Geometry check sheet. Reference: the model listing, model coordinates, mm. Face numbers are marked on the shaded views. A direction names the side the tool comes from. Give positions to 0.01 mm unless a question says otherwise; leave off trailing zeros. Loops run counter-clockwise (first coordinate to the right, second up) from the corner with the lowest first, then second, coordinate; pieces in that order, holes last.
1. Cross-section at B-B, the plane z = 0. Record the cut outline in (x, y).
2. Go/stop test with flat-tipped pins: pin 1 Ø3 at (x, y) = (9, 2) entering from +Z; pin 2 Ø2.5 at (x, z) = (28, -1) entering from +Y; pin 3 Ø0.6 at (y, z) = (1.5, -5) entering from -X. Record where each tip stops, or that it passes through.
3. Tool access check on the marked faces 1, 2 and 3. Record the directions out of +Z, -Z, +X, -X, +Y, -Y that give a thin tool (end or side, any length) a straight path to the whole face; none if there is none.
4. Material ranges on L1, parallel to X at y = -1, z = 0.25; L2, parallel to Z at x = 18, y = 2.5; L3, parallel to Y at x = 10, z = 3.25, recorded low to high.
5. Cross-section at C-C, the plane y = 4. Record the cut outline in (x, z).
6. Release check for a two-part mould opening along X. For the marked faces 4, 5 and 6 record: +X half, -X half, draft (parallel to the pull), parting line (faces both ways), or undercut.
7. Cross-section at A-A, the plane x = 25. Record the cut outline in (y, z).
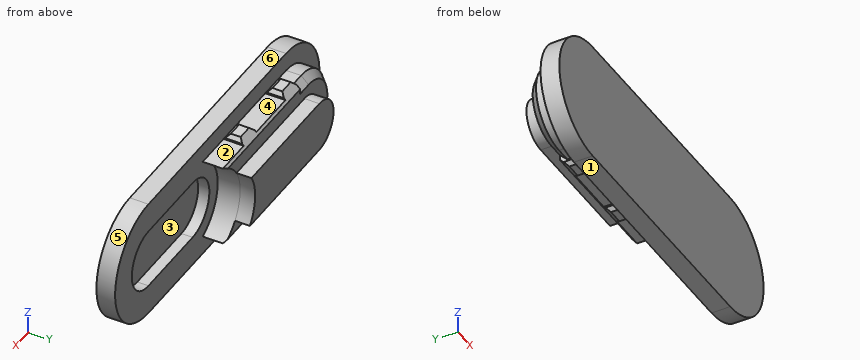
from build123d import *

# Parameters (mm, degrees)
EXTRUDE_1_DEPTH          = 3
EXTRUDE_2_DEPTH          = 2.5
CUT_EXTRUDE_1_DEPTH      = 1.5
EXTRUDE_3_DEPTH          = 2
SKETCH_5_W               = 3
SKETCH_5_H               = 0.7
EXTRUDE_4_DEPTH          = 3
CHAMFER_1_SIZE           = 1
CHAMFER_START            = -5.499796234
CHAMFER_2_DEPTH          = 7.499796234
CHAMFER_2_2_ANGLE        = 180
CHAMFER_3_SIZE           = 0.5
CUT_EXTRUDE_2_DEPTH      = 43.071367936
CUT_EXTRUDE_2_DEPTH_BACK = 43.071367936


with BuildPart() as part:
    # 草图1 → 凸台-拉伸1 (new body)
    with BuildSketch(Plane(origin=(0, 0, 0), x_dir=(1, 0, 0), z_dir=(0, 1, 0))):
        with BuildLine():
            Line((0, 5.5), (20.002084238, 5.5))
            ThreePointArc((20.002084238, 5.5), (16.4, 0), (20.002084238, -5.5))
            Line((20.002084238, -5.5), (0, -5.5))
            ThreePointArc((0, -5.5), (-5.5, 0), (0, 5.5))
        make_face()
    extrude(amount=EXTRUDE_1_DEPTH)

    # 草图2 → 凸台-拉伸2 (add)
    with BuildSketch(Plane.XZ):
        with BuildLine():
            Line((0, 8), (33, 8))
            ThreePointArc((33, 8), (41, 0), (33, -8))
            Line((33, -8), (0, -8))
            ThreePointArc((0, -8), (-8, 0), (0, 8))
        make_face()
    extrude(amount=EXTRUDE_2_DEPTH)

    # 草图3 → 切除-拉伸1 (cut)
    with BuildSketch(Plane(origin=(0, 0, 0), x_dir=(1, 0, 0), z_dir=(0, 1, 0))):
        with BuildLine():
            Line((22.4, 4), (33, 4))
            ThreePointArc((33, 4), (37, 0), (33, -4))
            Line((33, -4), (22.4, -4))
            ThreePointArc((22.4, -4), (18.4, 0), (22.4, 4))
        make_face()
    extrude(amount=-CUT_EXTRUDE_1_DEPTH, mode=Mode.SUBTRACT)

    # 草图4 → 凸台-拉伸3 (add)
    with BuildSketch(Plane(origin=(0, 3, 0), x_dir=(1, 0, 0), z_dir=(0, 1, 0))):
        with BuildLine():
            Line((1, 3.65), (17.637910123, 3.65))
            ThreePointArc((17.637910123, 3.65), (16.407686099, 0.30360189), (17.293386641, -3.15))
            Line((17.293386641, -3.15), (1, -3.15))
            ThreePointArc((1, -3.15), (-2.4, 0.25), (1, 3.65))
        make_face()
    extrude(amount=EXTRUDE_3_DEPTH)

    # 草图5 → 凸台-拉伸4 (add)
    with BuildSketch(Plane(origin=(0, 0, 0), x_dir=(1, 0, 0), z_dir=(0, 1, 0))):
        with Locations((3.5, 5.85)):
            Rectangle(SKETCH_5_W, SKETCH_5_H)
        with Locations((13.5, 5.85)):
            Rectangle(SKETCH_5_W, SKETCH_5_H)
        with Locations((13.5, -5.85)):
            Rectangle(SKETCH_5_W, SKETCH_5_H)
        with Locations((3.5, -5.85)):
            Rectangle(SKETCH_5_W, SKETCH_5_H)
    extrude(amount=EXTRUDE_4_DEPTH)

    # 倒角1
    chamfer_1_edges = [part.edges().sort_by_distance(p)[0] for p in [
        (3.5, 3, -6.2),
        (3.5, 3, 6.2),
    ]]
    chamfer(chamfer_1_edges, length=CHAMFER_1_SIZE)

    # 倒角2: read off the stored shape, not the designer's step
    # 倒角2 outline → 倒角2 (cut)
    with BuildSketch(Plane.YZ.offset(CHAMFER_START)):
        Polygon((3, -5.2), (3, -4.5), (2, -5.5), (2.7, -5.5), align=None)
        Polygon((2, 5.5), (3, 4.5), (3, 5.2), (2.7, 5.5), align=None)
    extrude(amount=CHAMFER_2_DEPTH, mode=Mode.SUBTRACT)

    # Chamfer 2 2 outline → Chamfer 2 2 (revolve, cut)
    with BuildSketch(Plane(origin=(0, 0, 0), x_dir=(0, 0, -1), z_dir=(1, 0, 0))):
        Polygon((5.5, 3), (4.5, 3), (5.5, 2), align=None)
    revolve(axis=Axis((0, 0, 0), (0, 1, 0)), revolution_arc=CHAMFER_2_2_ANGLE, mode=Mode.SUBTRACT)

    # 倒角3
    chamfer_3_edges = [part.edges().sort_by_distance(p)[0] for p in [
        (2, 1, -6.2),
        (5, 1, -6.2),
        (12, 1, -6.2),
        (15, 1, -6.2),
        (15, 1, 6.2),
        (12, 1, 6.2),
        (5, 1, 6.2),
        (2, 1, 6.2),
    ]]
    chamfer(chamfer_3_edges, length=CHAMFER_3_SIZE)

    # 草图6 → 切除-拉伸2 (cut, two sides: drawn at the far end of the back side and taken through both)
    with BuildSketch(Plane(origin=(0, 0, 0), x_dir=(0, 0, -1), z_dir=(1, 0, 0)).offset(-CUT_EXTRUDE_2_DEPTH_BACK)):
        Polygon((-5.5, 0), (-6.2, 0.7), (-6.2, 0), align=None)
        Polygon((5.5, 0), (6.2, 0), (6.2, 0.7), align=None)
    extrude(amount=CUT_EXTRUDE_2_DEPTH + CUT_EXTRUDE_2_DEPTH_BACK, mode=Mode.SUBTRACT)


solid = part.part
Result:
1. outline: (-8, -2.5) - (41, -2.5) - (41, 0) - (37, 0) - (37, -1.5) - (18.4, -1.5) - (18.4, 0) - (16.4, 0) - (16.4, 5) - (-2.39, 5) - (-2.39, 3) - (-4.5, 3) - (-5.5, 2) - (-5.5, 0) - (-8, 0) - close
2. pin 1: stops at z = 5.5
2. pin 2: stops at y = -1.5
2. pin 3: stops at x = -2.86
3. face 1: -Z, +X, -X, +Y, -Y
3. face 2: +Z, +X, +Y
3. face 3: +Y
4. L1: x = -8 to 18.41, 36.99 to 41
4. L2: z = -5.5 to -4.08, 4.08 to 5.5
4. L3: y = -2.5 to 3
5. outline: (1, -3.65) - (17.64, -3.65) arc R6 cw to (17.29, 3.15) - (1, 3.15) arc R3.4 ccw to start
6. face 4: undercut
6. face 5: +X half
6. face 6: draft
7. outline: (-2.5, -8) - (0, -8) - (0, -4) - (-1.5, -4) - (-1.5, 4) - (0, 4) - (0, 8) - (-2.5, 8) - close
